from build123d import *

# Parameters (mm, degrees)
CROQUIS1_R              = 110
SALIENTE_EXTRUIR1_DEPTH = 10
CROQUIS2_R              = 3.862102747
CROQUIS2_R_2            = 4
CORTAR_EXTRUIR1_DEPTH   = 10
CROQUIS3_R              = 60
CORTAR_EXTRUIR2_DEPTH   = 10
CROQUIS4_R              = 3.25
CORTAR_EXTRUIR3_DEPTH   = 10
CROQUIS5_R              = 7.35
CORTAR_EXTRUIR4_DEPTH   = 2
CROQUIS7_R              = 1.5
CORTAR_EXTRUIR5_DEPTH   = 10


with BuildPart() as part:
    # Croquis1 → Saliente-Extruir1 (new body)
    with BuildSketch(Plane(origin=(0, 0, 0), x_dir=(1, 0, 0), z_dir=(0, 1, 0))):
        with Locations(Location((0, 0, 0), (0, 0, 270))):
            Circle(CROQUIS1_R)
    extrude(amount=SALIENTE_EXTRUIR1_DEPTH)

    # Croquis2 → Cortar-Extruir1 (cut)
    with BuildSketch(Plane(origin=(0, 10, 0), x_dir=(1, 0, 0), z_dir=(0, 1, 0))):
        with Locations(Location((0, 100, 0), (0, 0, 270))):
            Circle(CROQUIS2_R)
        with Locations(Location((-100, 0, 0), (0, 0, 270))):
            Circle(CROQUIS2_R_2)
        with Locations(Location((0, -100, 0), (0, 0, 270))):
            Circle(CROQUIS2_R_2)
        with Locations(Location((100, 0, 0), (0, 0, 270))):
            Circle(CROQUIS2_R_2)
        with Locations(Location((-70.710678119, 70.710678119, 0), (0, 0, 270))):
            Circle(CROQUIS2_R_2)
        with Locations(Location((70.710678119, 70.710678119, 0), (0, 0, 270))):
            Circle(CROQUIS2_R_2)
        with Locations(Location((70.710678119, -70.710678119, 0), (0, 0, 270))):
            Circle(CROQUIS2_R_2)
        with Locations(Location((-70.710678119, -70.710678119, 0), (0, 0, 270))):
            Circle(CROQUIS2_R_2)
    extrude(amount=-CORTAR_EXTRUIR1_DEPTH, mode=Mode.SUBTRACT)

    # Croquis3 → Cortar-Extruir2 (cut)
    with BuildSketch(Plane(origin=(0, 10, 0), x_dir=(1, 0, 0), z_dir=(0, 1, 0))):
        with Locations(Location((0, 0, 0), (0, 0, 270))):
            Circle(CROQUIS3_R)
    extrude(amount=-CORTAR_EXTRUIR2_DEPTH, mode=Mode.SUBTRACT)

    # Croquis4 → Cortar-Extruir3 (cut)
    with BuildSketch(Plane(origin=(0, 10, 0), x_dir=(1, 0, 0), z_dir=(0, 1, 0))):
        with Locations(Location((89.254735783, -35.349570581, 0), (0, 0, 270))):
            Circle(CROQUIS4_R)
        with Locations(Location((-35.349570581, -89.254735783, 0), (0, 0, 270))):
            Circle(CROQUIS4_R)
        with Locations(Location((-89.254735783, 35.349570581, 0), (0, 0, 270))):
            Circle(CROQUIS4_R)
        with Locations(Location((35.349570581, 89.254735783, 0), (0, 0, 270))):
            Circle(CROQUIS4_R)
    extrude(amount=-CORTAR_EXTRUIR3_DEPTH, mode=Mode.SUBTRACT)

    # Croquis5 → Cortar-Extruir4 (cut)
    with BuildSketch(Plane(origin=(0, 10, 0), x_dir=(1, 0, 0), z_dir=(0, 1, 0))):
        with Locations(Location((91.046524442, 38.842229875, 0), (0, 0, 270))):
            Circle(CROQUIS5_R)
        with Locations(Location((38.842229875, -91.046524442, 0), (0, 0, 270))):
            Circle(CROQUIS5_R)
        with Locations(Location((-91.046524442, -38.842229875, 0), (0, 0, 270))):
            Circle(CROQUIS5_R)
        with Locations(Location((-38.842229875, 91.046524442, 0), (0, 0, 270))):
            Circle(CROQUIS5_R)
    extrude(amount=-CORTAR_EXTRUIR4_DEPTH, mode=Mode.SUBTRACT)

    # Croquis7 → Cortar-Extruir5 (cut)
    with BuildSketch(Plane(origin=(0, 10, 0), x_dir=(1, 0, 0), z_dir=(0, 1, 0))):
        with Locations(Location((-38.842229875, 91.046524442, 0), (0, 0, 270))):
            Circle(CROQUIS7_R)
        with Locations(Location((91.046524442, 38.842229875, 0), (0, 0, 270))):
            Circle(CROQUIS7_R)
        with Locations(Location((38.842229875, -91.046524442, 0), (0, 0, 270))):
            Circle(CROQUIS7_R)
        with Locations(Location((-91.046524442, -38.842229875, 0), (0, 0, 270))):
            Circle(CROQUIS7_R)
    extrude(amount=-CORTAR_EXTRUIR5_DEPTH, mode=Mode.SUBTRACT)


solid = part.part
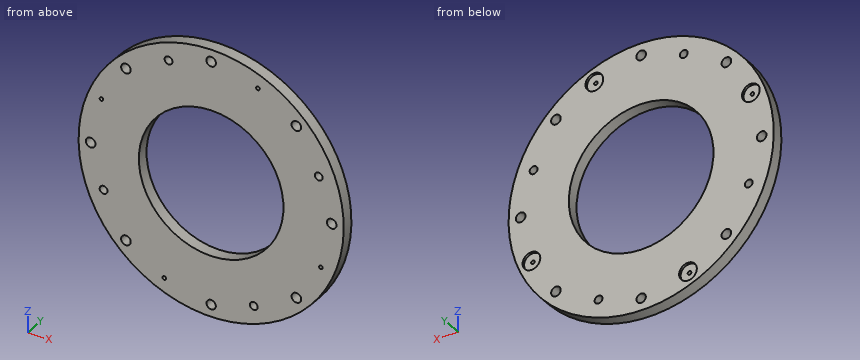
The model under review builds one solid part; all positions refer to its coordinate system, in mm. Give positions to 0.01 mm unless a question says otherwise; leave off trailing zeros. Loops run counter-clockwise (first coordinate to the right, second up) from the corner with the lowest first, then second, coordinate; pieces in that order, holes last. Notation, with made-up numbers: (-2, 53.25) -> (7, 53.25) arc R21 ccw to (7, 73.25) -> close; hole circle Ø9 at (62.25, 39.25). An arc over 180 degrees is marked (long way). Answer as a JSON object with one key per item and string values. Group by question number.
Q1. Insertion check: pin 1 (1 mm diameter, centred on y = 7, z = -66.5, fed in from -X); pin 2 (2.5 mm diameter, centred on x = -91.05, z = 38.84, fed in from -Y); pin 3 (2 mm diameter, centred on x = -73, y = 7, fed in from -Z); pin 4 (3 mm diameter, centred on x = -70.5, y = 3, fed in from +Z). Each pin has a flat end and moves straight along its axis. Give the tip position at first contact, or say it passes through.
Q2. Take a section at D-D (y = 6.5). State how many separate pieces and enclosed holes the cut face has, plus the area to 3 significant figures.
Q3. Take a section at A-A (x = 0). Write out the cut boundary in (y, z), plus the area to 3 significant figures.
Q4. Take a section at C-C (x = -56). Write out the cut boundary in (y, z).
Q5. Take a section at B-B (z = -19). Write out the cut boundary in (x, y), plus the area to 3 significant figures.
Q6. Wall thickness on line 1 along X through (y, z) = (4.5, -37); line 2 along X through (y, z) = (9.75, -90); line 3 along Z through (x, y) = (41, 8.75): over which ranges is each line inside the solid? List them lowest first.
Answer below:
{
 "1": {"pin 1": "stops at x = -88", "pin 2": "passes through", "pin 3": "stops at z = -83.16", "pin 4": "stops at z = 85.67"},
 "2": {"separate pieces": "1", "enclosed holes": "17", "area": "26,100 mm2"},
 "3": {"outline": "(0, -110) -> (10, -110) -> (10, -103.86) -> (0, -103.86) -> close; (0, -96.14) -> (10, -96.14) -> (10, -60) -> (0, -60) -> close; (0, 60) -> (10, 60) -> (10, 96) -> (0, 96) -> close; (0, 104) -> (10, 104) -> (10, 110) -> (0, 110) -> close", "area": "843 mm2"},
 "4": {"outline": "(0, -94.68) -> (10, -94.68) -> (10, -21.54) -> (0, -21.54) -> close; (0, 21.54) -> (10, 21.54) -> (10, 94.68) -> (0, 94.68) -> close"},
 "5": {"outline": "(-108.35, 0) -> (-56.91, 0) -> (-56.91, 10) -> (-108.35, 10) -> close; (56.91, 0) -> (108.35, 0) -> (108.35, 10) -> (56.91, 10) -> close", "area": "1,030 mm2"},
 "6": {"line 1": "x = -103.59 to -92.05, -86.45 to -47.23, 47.23 to 103.59", "line 2": "x = -63.25 to -46.12, -31.57 to 32.19, 38.51 to 63.25", "line 3": "z = -102.07 to -43.81, 43.81 to 84.02, 98.07 to 102.07"}
}
